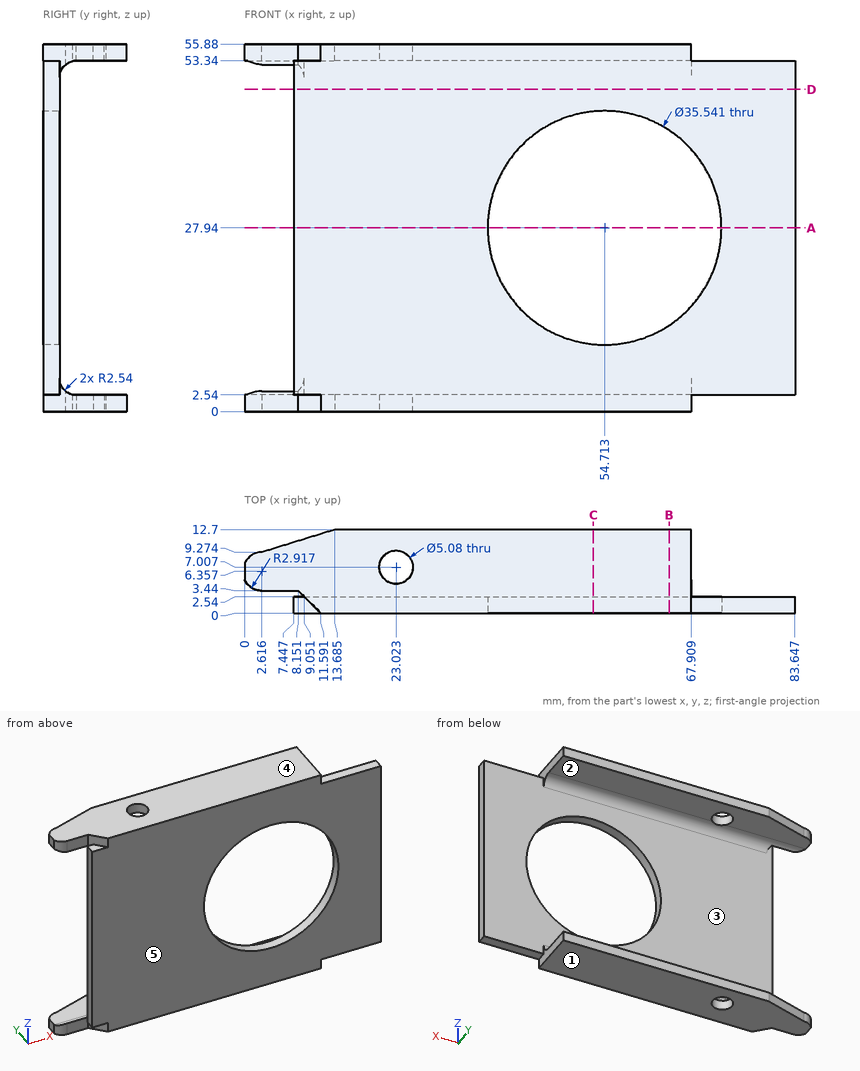
Answer from the drawing. Dimensions are ordinates in mm from the lowest x, y and z of the part. A direction names the side the tool comes from. Round coordinates to 2 decimals unless told otherwise and drop trailing zeros. Write each loop counter-clockwise with the first axis right and the second up, starting at its lowest first coordinate (ties: lowest second). Pieces come first, ordered by that corner, then holes. Notation, with made-up numbers: (8.5, 15.5) -> (24.5, 15.5) arc R17 ccw to (24.5, 28.5) -> close; hole circle Ø3 at (50.5, -5). An arc over 180 degrees is marked (long way). Write each question's results on one line, items separated by ' | '.
1) The part is cut by section C-C (x = 53). Write down the section's boundary in (y, z).
Findings:
outline: (0, 0) -> (12.7, 0) -> (12.7, 2.54) -> (5.08, 2.54) arc R2.54 cw to (2.54, 5.08) -> (2.54, 10.25) -> (0, 10.25) -> close; (0, 45.63) -> (2.54, 45.63) -> (2.54, 50.8) arc R2.54 cw to (5.08, 53.34) -> (12.7, 53.34) -> (12.7, 55.88) -> (0, 55.88) -> close
2) For a pull along Z with two mould halves and no side action, classify the marked faces 3, 4 and 5 as +Z half, -Z half, draft (parallel to the pull), parting line (faces both ways), or undercut.
Findings:
face 3: undercut | face 4: +Z half | face 5: draft
3) The part is cut by section D-D (z = 49). Write down the section's boundary in (x, y).
Findings:
outline: (7.45, 0) -> (83.65, 0) -> (83.65, 2.54) -> (7.45, 2.54) -> close
4) Flat-ended cylindrical pins translate along their axes: pin 1 (0.9 mm diameter, centred on x = 4, z = 2.5, fed in from -Y); pin 2 (2 mm diameter, centred on x = 9, y = 1, fed in from -Z); pin 3 (5.5 mm diameter, centred on y = 6, z = 54, fed in from +X); pin 4 (4.5 mm diameter, centred on x = 23.02, y = 7.01, fed in from -Z). Find the tip coordinate at first contact, or state that the pin passes through.
Findings:
pin 1: stops at y = 3.44 | pin 2: stops at z = 2.54 | pin 3: stops at x = 67.91 | pin 4: passes through
5) The part is cut by section A-A (z = 27.94). Write down the section's boundary in (x, y).
Findings:
outline: (7.45, 0) -> (36.94, 0) -> (36.94, 2.54) -> (7.45, 2.54) -> close; (72.48, 0) -> (83.65, 0) -> (83.65, 2.54) -> (72.48, 2.54) -> close
6) Which of the six approach directions +Z, -Z, +X, -X, +Y, -Y give full straight-line access (tool end or side, diameter ignored) to the marked faces 1 and 2?
Findings:
face 1: -Z, +X, -X, +Y, -Y | face 2: +X, -X, +Y
7) The part is cut by section B-B (x = 64.5). Write down the section's boundary in (y, z), and give its area (3 significant figures).
Findings:
outline: (0, 0) -> (12.7, 0) -> (12.7, 2.54) -> (5.08, 2.54) arc R2.54 cw to (2.54, 5.08) -> (2.54, 13.11) -> (0, 13.11) -> close; (0, 42.77) -> (2.54, 42.77) -> (2.54, 50.8) arc R2.54 cw to (5.08, 53.34) -> (12.7, 53.34) -> (12.7, 55.88) -> (0, 55.88) -> close | area: 121 mm²
8) Consider line 1 along X through (y, z) = (1.4, 27.94); line 2 along Z through (x, y) = (41, 7.5); line 3 along Y through (x, z) = (69, 52.5). Determine where each line is inside the solid, lowest interval first. Write a range as [from, to].
Findings:
line 1: x = [7.45, 36.94], [72.48, 83.65] | line 2: z = [0, 2.54], [53.34, 55.88] | line 3: y = [0, 2.54]
